Check sheet for the modelled part. Datum: model origin and axes. Units: mm. A direction names the side the tool comes from. Round coordinates to 2 decimals unless told otherwise and drop trailing zeros. Write each loop counter-clockwise with the first axis right and the second up, starting at its lowest first coordinate (ties: lowest second). Pieces come first, ordered by that corner, then holes. Notation, with made-up numbers: (-36.75, 72) - (-31.75, 72) arc R7 cw to (-31.75, 77) - close; hole circle Ø11 at (-9, -37). An arc over 180 degrees is marked (long way). Answer as a JSON object with one key per item and string values. Group by question number.
Item 1: Release check for a two-part mould opening along Z. For faces 4 (the flat face through (-1, 16, -29.5)), 5 (the flat face through (-1, 14, 32.5)), 6 (the flat face through (-26, 28, -31)) record: pulls with the +Z half, pulls with the -Z half, needs draft (parallel to the pull), parting line crosses it, or undercut.
Item 2: Sectioned sample at C-C on y = 20. Record the boundary of the cut face in (x, z), plus the area to 3 significant figures.
Item 3: Sectioned sample at A-A on y = 10.5. Record the boundary of the cut face in (x, z), plus the area to 3 significant figures.
Item 4: Gauge pin test, flat ends, axial feed: P1, Ø1.2, axis at x = -85, z = -31, coming from the +Y side; P2, Ø1.5, axis at x = 22, z = 0, coming from the +Y side. Record the tip position at first contact, or that the pin passes through.
Item 5: Set-up check for faces 1 (the flat face through (86, 23.5, -1)), 2 (the flat face through (-87, 14, 0)), 3 (the flat face through (-1, 16, 29.5)): record each of +Z, -Z, +X, -X, +Y, -Y from which the full face is reachable in a straight line by a thin tool's end or side.
Item 6: Sectioned sample at B-B on z = 13. Record the boundary of the cut face in (x, y).
Item 7: Sectioned sample at D-D on x = -73. Record the boundary of the cut face in (y, z).
Item 8: Thickness scan on line 1 (X direction, y = 25.2, z = -31); line 2 (Z direction, x = -85.5, y = 26.4); line 3 (Z direction, x = 21.5, y = 11). Record the ranges inside material, lowest first.
```python
from build123d import *

# Parameters (mm, degrees)
SKETCH1_W           = 174
SKETCH1_H           = 65
BOSS_EXTRUDE1_DEPTH = 5
SKETCH2_W           = 174
SKETCH2_H           = 65
SKETCH2_W_2         = 168
SKETCH2_H_2         = 59
BOSS_EXTRUDE2_DEPTH = 23
CUT_EXTRUDE1_DEPTH  = 23
SKETCH4_R           = 1.25
CUT_EXTRUDE2_DEPTH  = 5


with BuildPart() as part:
    # Sketch1 → Boss-Extrude1 (new body)
    with BuildSketch(Plane(origin=(0, 0, 0), x_dir=(1, 0, 0), z_dir=(0, 1, 0))):
        Rectangle(SKETCH1_W, SKETCH1_H)
    extrude(amount=BOSS_EXTRUDE1_DEPTH)

    # Sketch2 → Boss-Extrude2 (add)
    with BuildSketch(Plane(origin=(0, 5, 0), x_dir=(1, 0, 0), z_dir=(0, 1, 0))):
        Rectangle(SKETCH2_W, SKETCH2_H)
        Rectangle(SKETCH2_W_2, SKETCH2_H_2, mode=Mode.SUBTRACT)
    extrude(amount=BOSS_EXTRUDE2_DEPTH)

    # Sketch3 → Cut-Extrude1 (cut)
    with BuildSketch(Plane(origin=(87, 0, 0), x_dir=(0, 0, -1), z_dir=(1, 0, 0))):
        with BuildLine():
            Line((-3, 23.5), (5, 23.5))
            ThreePointArc((5, 23.5), (8.5, 20), (5, 16.5))
            Line((5, 16.5), (-3, 16.5))
            ThreePointArc((-3, 16.5), (-6.5, 20), (-3, 23.5))
        make_face()
    extrude(amount=-CUT_EXTRUDE1_DEPTH, mode=Mode.SUBTRACT)

    # Sketch4 → Cut-Extrude2 (cut)
    with BuildSketch(Plane(origin=(0, 28, 0), x_dir=(1, 0, 0), z_dir=(0, 1, 0))):
        with Locations(Location((-85.5, 31, 0), (0, 0, 270))):
            Circle(SKETCH4_R)
        with Locations(Location((85.5, 31, 0), (0, 0, 270))):
            Circle(SKETCH4_R)
        with Locations(Location((85.5, -31, 0), (0, 0, 270))):
            Circle(SKETCH4_R)
        with Locations(Location((-85.5, -31, 0), (0, 0, 270))):
            Circle(SKETCH4_R)
    extrude(amount=-CUT_EXTRUDE2_DEPTH, mode=Mode.SUBTRACT)


solid = part.part
```
Completed:
{
 "1": {"face 4": "undercut", "face 5": "pulls with the +Z half", "face 6": "needs draft"},
 "2": {"outline": "(-87, -32.5) - (87, -32.5) - (87, -8.5) - (84, -8.5) - (84, -29.5) - (-84, -29.5) - (-84, 29.5) - (84, 29.5) - (84, 6.5) - (87, 6.5) - (87, 32.5) - (-87, 32.5) - close", "area": "1,350 mm²"},
 "3": {"outline": "(-87, -32.5) - (87, -32.5) - (87, 32.5) - (-87, 32.5) - close; hole (-84, -29.5) - (84, -29.5) - (84, 29.5) - (-84, 29.5) - close", "area": "1,400 mm²"},
 "4": {"P1": "y = 23", "P2": "y = 5"},
 "5": {"face 1": "+X", "face 2": "+Z, -Z, -X, +Y, -Y", "face 3": "+Y"},
 "6": {"outline": "(-87, 0) - (87, 0) - (87, 28) - (84, 28) - (84, 5) - (-84, 5) - (-84, 28) - (-87, 28) - close"},
 "7": {"outline": "(0, -32.5) - (28, -32.5) - (28, -29.5) - (5, -29.5) - (5, 29.5) - (28, 29.5) - (28, 32.5) - (0, 32.5) - close"},
 "8": {"line 1": "-87 to -86.75, -84.25 to 84.25, 86.75 to 87", "line 2": "-32.5 to -32.25, -29.75 to 29.75, 32.25 to 32.5", "line 3": "-32.5 to -29.5, 29.5 to 32.5"}
}
